Drawing for the job (mm, zero at the part's lowest x, y, z). A direction names the side the tool comes from. Coordinates: 2 decimals unless noted, no trailing zeros. Order: outer loops, then holes, each group sorted by start corner. A loop starts at its lowest first (then second) coordinate and runs counter-clockwise, first axis right, second up.
1) Tool access for the marked faces 1, 2 and 3: list every direction of +Z, -Z, +X, -X, +Y, -Y with a clear straight run to the whole face (end or side of a thin tool).
2) Wall check: L1, parallel to Z at x = 20, y = 31; L2, parallel to Y at x = 48.5, z = 11.5; L3, parallel to Z at x = 41.5, y = 6.5. Give the ranges that are in metal, low to high.
3) Cut at B-B (z = 27.5). List the corners of the cut face in (x, y), and give its area (3 significant figures).
4) Cut at A-A (y = 34.5). List the corners of the cut face in (x, z), and give its area (3 significant figures).
5) Cut at C-C (x = 26). List the corners of the cut face in (y, z).
6) Pin check, flat tips, straight feed: pin 1 Ø10 at (y, z) = (24, 27.5) entering from +X; pin 2 Ø5 at (x, y) = (45, 32.5) entering from +Z; pin 3 Ø1.5 at (y, z) = (32.5, 12.5) entering from +X. Stop position of each tip, or through.
7) Mould opens along Z. For the marked faces 4, 5, 6 and 7 say: +Z half, -Z half, draft (parallel to the pull), parting line (faces both ways), or undercut.
8) Cut at D-D (y = 8). List the corners of the cut face in (x, z), and give its area (3 significant figures).
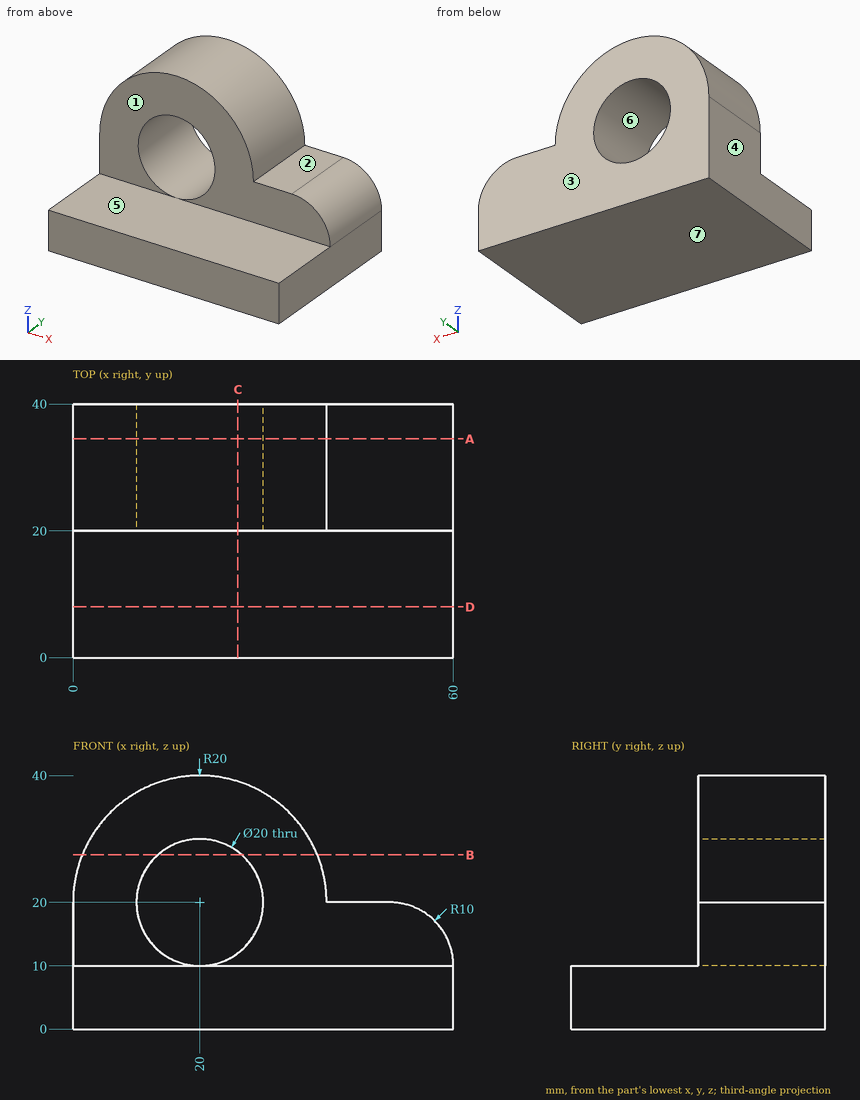
Geometry check:
1. face 1: +Z, +X, -X, -Y
1. face 2: +Z, +X, +Y, -Y
1. face 3: +Z, -Z, +X, -X, +Y
2. L1: z = 0 to 10, 30 to 40
2. L2: y = 20 to 40
2. L3: z = 0 to 10
3. outline: (1.46, 20) - (13.39, 20) - (13.39, 40) - (1.46, 40) - close; (26.61, 20) - (38.54, 20) - (38.54, 40) - (26.61, 40) - close
3. area: 477 mm2
4. outline: (0, 0) - (60, 0) - (60, 10) arc R10 ccw to (50, 20) - (40, 20) arc R20 ccw to (0, 20) - close; hole circle Ø20 at (20, 20)
4. area: 1,490 mm2
5. outline: (0, 0) - (40, 0) - (40, 12) - (20, 12) - (20, 10) - (0, 10) - close; (20, 28) - (40, 28) - (40, 39.08) - (20, 39.08) - close
6. pin 1: stops at x = 39.84
6. pin 2: stops at z = 20
6. pin 3: stops at x = 59.85
7. face 4: draft
7. face 5: +Z half
7. face 6: undercut
7. face 7: -Z half
8. outline: (0, 0) - (60, 0) - (60, 10) - (0, 10) - close
8. area: 600 mm2
